Work out the finished part from the listing and answer in its coordinate system (mm). A direction names the side the tool comes from. Round coordinates to 2 decimals unless told otherwise and drop trailing zeros. Order: outer loops, then holes, each group sorted by start corner. A loop starts at its lowest first (then second) coordinate and runs counter-clockwise, first axis right, second up. Notation, with made-up numbers: (73, 5.5) - (126, 5.5) arc R8 cw to (126, 17.5) - close; hole circle Ø4 at (-28.75, -18). An arc over 180 degrees is marked (long way). Put each result on its own line as item: value.
```python
from build123d import *

# Parameters (mm, degrees)
SKETCH_1_W          = 6
SKETCH_1_H          = 4
EXTRUDE_1_DEPTH     = 5
SKETCH_2_R          = 0.5
CUT_EXTRUDE_1_DEPTH = 5
EXTRUDE_2_DEPTH     = 0.5
EXTRUDE_3_DEPTH     = 1
SKETCH_5_R          = 0.45
CUT_EXTRUDE_2_DEPTH = 6
FILLET_1_R          = 1


with BuildPart() as part:
    # Sketch 1 → Extrude 1 (new body)
    with BuildSketch(Plane.XY):
        Rectangle(SKETCH_1_W, SKETCH_1_H)
    extrude(amount=EXTRUDE_1_DEPTH)

    # Sketch 2 → Cut-Extrude 1 (cut)
    with BuildSketch(Plane(origin=(0, 0, 0), x_dir=(-1, 0, 0), z_dir=(0, 0, -1))):
        with Locations((-1.2, 0)):
            Circle(SKETCH_2_R)
        with Locations((1.2, 0)):
            Circle(SKETCH_2_R)
    extrude(amount=-CUT_EXTRUDE_1_DEPTH, mode=Mode.SUBTRACT)

    # Sketch 3 → Extrude 2 (add)
    with BuildSketch(Plane(origin=(0, 2, 0), x_dir=(1, 0, 0), z_dir=(0, 1, 0))):
        Polygon((-0.909925586, 0), (0, -2.5), (0.909925586, 0), align=None)
        Polygon((0.909925586, 0), (0, -2.5), (2.090074414, -2.5), (3, 0), align=None)
        Polygon((-2.090074414, -2.5), (0, -2.5), (-0.909925586, 0), (-3, 0), align=None)
        Polygon((-3, 0), (-0.909925586, 0), (-2.638633265, 4.749585314), (-4.484215418, 4.077848346), align=None)
        Polygon((2.638633265, 4.749585314), (0.909925586, 0), (3, 0), (4.484215418, 4.077848346), align=None)
    extrude(amount=EXTRUDE_2_DEPTH)

    # Sketch 3_7 → Extrude 3 (add)
    with BuildSketch(Plane(origin=(0, 2, 0), x_dir=(1, 0, 0), z_dir=(0, 1, 0))):
        Polygon((-3, 0), (-0.909925586, 0), (-2.638633265, 4.749585314), (-4.484215418, 4.077848346), align=None)
        Polygon((2.638633265, 4.749585314), (0.909925586, 0), (3, 0), (4.484215418, 4.077848346), align=None)
        Polygon((-2.090074414, -2.5), (0, -2.5), (-0.909925586, 0), (-3, 0), align=None)
        Polygon((0.909925586, 0), (0, -2.5), (2.090074414, -2.5), (3, 0), align=None)
    extrude(amount=-EXTRUDE_3_DEPTH)

    # Sketch 5 → Cut-Extrude 2 (cut)
    with BuildSketch(Plane(origin=(-1.835148753, 0, -5.04202976), x_dir=(-0.939692621, 0, 0.342020143), z_dir=(-0.342020143, 0, -0.939692621))):
        with Locations((1.83706411, 2.5)):
            Circle(SKETCH_5_R)
    cut_extrude_2 = extrude(amount=-CUT_EXTRUDE_2_DEPTH, mode=Mode.SUBTRACT)

    # Mirror 1: Cut-Extrude 2 across plane
    add(cut_extrude_2.mirror(Plane(origin=(0, 0, 0), x_dir=(0, 0, 1), z_dir=(1, 0, 0))), mode=Mode.SUBTRACT)

    # Fillet 1
    fillet_1_edges = [part.edges().sort_by_distance(p)[0] for p in [
        (-3, 0, 5),
        (0, -2, 5),
        (3, 0, 5),
        (0, 2, 5),
    ]]
    fillet(fillet_1_edges, radius=FILLET_1_R)


solid = part.part
```
1) For a pull along Y with two mould halves and no side action, classify faces 1 (the cylindrical face through (-2.54, 2.05, -1.64)), 2 (the cylindrical face through (-1.662, -0.192, 2.465)), 3 (the flat face through (-3, 1, -2)) as pulls with the +Y half, pulls with the -Y half, needs draft (parallel to the pull), parting line crosses it, or undercut.
Findings below:
face 1: pulls with the +Y half
face 2: undercut
face 3: pulls with the -Y half
2) A cutting plane is placed at A-A on y = 0.3. Write down the section's boundary in (x, z), then the cut area to 3 significant figures.
Findings below:
outline: (-3, 0) - (-1.6, 0) - (-1.6, 5) - (-2, 5) arc R1 ccw to (-3, 4) - close; (-0.8, 0) - (0.8, 0) - (0.8, 5) - (-0.8, 5) - close; (1.6, 0) - (3, 0) - (3, 4) arc R1 ccw to (2, 5) - (1.6, 5) - close
area: 21.6 mm2
3) A cutting plane is placed at D-D on y = 0.85. Write down the section's boundary in (x, z), then the cut area to 3 significant figures.
Findings below:
outline: (-3, 0) - (3, 0) - (3, 4) arc R1 ccw to (2, 5) - (-2, 5) arc R1 ccw to (-3, 4) - close
area: 29.6 mm2
4) A cutting plane is placed at B-B on x = 0.5. Write down the section's boundary in (y, z).
Findings below:
outline: (-2, 0) - (2.5, 0) - (2.5, 2.5) - (2, 2.5) - (2, 4) arc R1 ccw to (1, 5) - (-1, 5) arc R1 ccw to (-2, 4) - close
5) Straight lines are drawn through the part: L1, parallel to Y at x = -1.2, z = 2.55; L2, parallel to Y at x = -1.2, z = 1.95; L3, parallel to X at y = 0.4, z = 1.25. For each, find the intervals that lie inside material, in ascending order. Write a range as from..to.
Findings below:
L1: y = -2..-0.5, 0.5..2
L2: y = -2..-0.5, 0.5..2.5
L3: x = -3..-1.5, -0.9..0.9, 1.5..3
6) Given pin 1 Ø0.6 at (x, y) = (-0.5, 2) entering from +Z; pin 2 Ø2 at (y, z) = (0.5, 2.5) entering from +X; pin 3 Ø3 at (x, z) = (2.5, -2) entering from -Y, each flat-ended and moving along its own axis, determine where each tip first touches the part or whether it passes through.
Findings below:
pin 1: stops at z = 4.71
pin 2: stops at x = 3
pin 3: stops at y = 1
7) A cutting plane is placed at C-C on z = 3. Write down the section's boundary in (x, y), then the cut area to 3 significant figures.
Findings below:
outline: (-3, -2) - (3, -2) - (3, 2) - (-3, 2) - close; hole circle Ø1 at (-1.2, 0); hole circle Ø1 at (1.2, 0)
area: 22.4 mm2
8) For faces 4 (the flat face through (-3, 0, 2)), 5 (the flat face through (0, -2, 2)), 6 (the flat face through (-1.76, 1.76, -2.34)), 7 (the flat face through (3, 0, 2)), 8 (the flat face through (0, 0, 0)), determine the directions among +Z, -Z, +X, -X, +Y, -Y from which every point of the face is accessible in a straight line to the end or side of a thin tool.
Findings below:
face 4: +Z, -X, +Y, -Y
face 5: +Z, -Z, +X, -X, -Y
face 6: -Z, +Y, -Y
face 7: +Z, +X, +Y, -Y
face 8: -Z, -Y
